Source: CAD feature listing. Evaluate the final solid. Frame: model axes, mm. A direction names the side the tool comes from. Give positions to 0.01 mm unless a question says otherwise; leave off trailing zeros. Order: outer loops, then holes, each group sorted by start corner. A loop starts at its lowest first (then second) coordinate and runs counter-clockwise, first axis right, second up. Notation, with made-up numbers: M 23.25,5.5 L 37.25,5.5 A23 ccw 37.25,29.5 Z; hole C 14.25,9.5 d9. An arc over 180 degrees is marked long. Answer in a Markdown table with one row per item. Add a question column.
(1) Section query A-A, the plane z = 2. Return loops of the section in (x, y), plus the area to 3 significant figures.
(2) Section query B-B, the plane z = 5. Return loops of the section in (x, y).
(3) Set-up query: faces 1 (the face through (11.16, 9.36, 2.23)), 2 (the face through (-11, -11, 3.5)), 3 (the face through (11.33, 9.87, 0.49)), 4 (the face through (0, -14, 0)). Return all of +Z, -Z, +X, -X, +Y, -Y with unobstructed straight access to the full face (end or side cutting, diameter ignored); none if empty.
(4) Mould query, pull axis X, two halves, no side actions, for faces 5 (the face through (-16, -11, 9.5)), 6 (the face through (20.03, 6.31, 5.19)), 7 (the face through (-11.16, -9.36, 2.23)). Classes: pulls with the +X half, pulls with the -X half, needs draft (parallel to the pull), parting line crosses it, or undercut.
(5) Pin query (flat end, axial travel): P1, Ø4, axis at x = -3.5, y = 16, coming from the +Z side; P2, Ø1.8, axis at x = -2, z = 5, coming from the +Y side; P3, Ø3, axis at x = -7.5, z = 6, coming from the +Y side; P4, Ø19, axis at x = -10.5, y = -10, coming from the +Z side. Return the tip coordinate at first contact, or that it passes through.
(6) Material intervals for line 1 along Y through (x, z) = (0, 8.15); line 2 along Y through (x, z) = (-8, 8.25); line 3 along X through (y, z) = (-3, 9.25), sorted ascending.
from build123d import *

# Parameters (mm, degrees)
F0_R         = 21
F1_DEPTH     = 3
F2_R         = 21
F3_DEPTH     = 0.5
F4_R         = 21
F5_DEPTH     = 3.5
F6_R         = 21
F6_R_2       = 19
F7_DEPTH     = 2.5
F8_SIZE      = 1
F9_T6_DEPTH  = 12.3424053326
F9_T11_DEPTH = 19.8242698458
F9_T17_DEPTH = 12.3424053326
F9_T20_ANGLE = 104.7950367117
F9_T24_DEPTH = 12.3424053326
F9_T29_DEPTH = 19.8242698458
F9_T35_DEPTH = 12.3424053326
F9_T38_ANGLE = 104.7950367117
F9_T43_DEPTH = 12.3424053326
F9_T47_DEPTH = 19.8242698458
F9_T54_DEPTH = 19.8242698458
F9_T58_DEPTH = 12.3424053326
F9_T65_DEPTH = 12.3424053326
F9_T69_DEPTH = 19.8242698458
F9_T76_DEPTH = 19.8242698458
F9_T80_DEPTH = 12.3424053326


# Not quite as in the source:
# - a fillet or chamfer that OpenCascade refuses, or shapes differently, is made with other operations: its cross-section is extruded or revolved along the edge and cut away or added


with BuildPart() as f1:
    # F0 (on Top) → F1 (new body)
    with BuildSketch(Plane.XY):
        Circle(F0_R)
        with BuildLine():
            Line((-15.0814358373, 6.3381057238), (-7.340451935, 12.3))
            Line((-7.340451935, 12.3), (7.340451935, 12.3))
            Line((7.340451935, 12.3), (15.0814358373, 6.3381057238))
            ThreePointArc((15.0814358373, 6.3381057238), (18.2, 0), (15.0814358373, -6.3381057238))
            Line((15.0814358373, -6.3381057238), (7.340451935, -12.3))
            Line((7.340451935, -12.3), (-7.340451935, -12.3))
            Line((-7.340451935, -12.3), (-15.0814358373, -6.3381057238))
            ThreePointArc((-15.0814358373, -6.3381057238), (-18.2, 0), (-15.0814358373, 6.3381057238))
        make_face(mode=Mode.SUBTRACT)
    extrude(amount=F1_DEPTH)

    # F2 (on face) → F3 (join)
    with BuildSketch(Plane.XY.offset(3)):
        Circle(F2_R)
        with BuildLine():
            Line((-15.0814358373, 6.3381057238), (-7.340451935, 12.3))
            Line((-7.340451935, 12.3), (-7.2180848246, 12.3))
            Line((-7.2180848246, 12.3), (-5.5458425084, 14.4712563576))
            ThreePointArc((-5.5458425084, 14.4712563576), (-3.0904049489, 16.4808755163), (0, 17.2))
            ThreePointArc((0, 17.2), (3.0904049489, 16.4808755163), (5.5458425084, 14.4712563576))
            Line((5.5458425084, 14.4712563576), (7.2180848246, 12.3))
            Line((7.2180848246, 12.3), (7.340451935, 12.3))
            Line((7.340451935, 12.3), (15.0814358373, 6.3381057238))
            ThreePointArc((15.0814358373, 6.3381057238), (17.3781434472, 3.5318913702), (18.2, 0))
            ThreePointArc((18.2, 0), (17.3781434472, -3.5318913702), (15.0814358373, -6.3381057238))
            Line((15.0814358373, -6.3381057238), (7.340451935, -12.3))
            Line((7.340451935, -12.3), (7.2180848246, -12.3))
            Line((7.2180848246, -12.3), (5.5458425084, -14.4712563576))
            ThreePointArc((5.5458425084, -14.4712563576), (3.0904049489, -16.4808755163), (0, -17.2))
            ThreePointArc((0, -17.2), (-3.0904049489, -16.4808755163), (-5.5458425084, -14.4712563576))
            Line((-5.5458425084, -14.4712563576), (-7.2180848246, -12.3))
            Line((-7.2180848246, -12.3), (-7.340451935, -12.3))
            Line((-7.340451935, -12.3), (-15.0814358373, -6.3381057238))
            ThreePointArc((-15.0814358373, -6.3381057238), (-17.3781434472, -3.5318913702), (-18.2, 0))
            ThreePointArc((-18.2, 0), (-17.3781434472, 3.5318913702), (-15.0814358373, 6.3381057238))
        make_face(mode=Mode.SUBTRACT)
    extrude(amount=F3_DEPTH)

    # F4 (on face) → F5 (join)
    with BuildSketch(Plane.XY.offset(3.5)):
        Circle(F4_R)
        with BuildLine():
            Line((-15.0814358373, 6.3381057238), (-7.340451935, 12.3))
            Line((-7.340451935, 12.3), (-7.2180848246, 12.3))
            Line((-7.2180848246, 12.3), (-5.5458425084, 14.4712563576))
            ThreePointArc((-5.5458425084, 14.4712563576), (-3.0904049489, 16.4808755163), (0, 17.2))
            ThreePointArc((0, 17.2), (12.8139825122, 12.529911728), (18.2, 0))
            ThreePointArc((18.2, 0), (17.3781434472, -3.5318913702), (15.0814358373, -6.3381057238))
            Line((15.0814358373, -6.3381057238), (7.340451935, -12.3))
            Line((7.340451935, -12.3), (7.2180848246, -12.3))
            Line((7.2180848246, -12.3), (5.5458425084, -14.4712563576))
            ThreePointArc((5.5458425084, -14.4712563576), (3.0904049489, -16.4808755163), (0, -17.2))
            ThreePointArc((0, -17.2), (-12.8139825122, -12.529911728), (-18.2, 0))
            ThreePointArc((-18.2, 0), (-17.3781434472, 3.5318913702), (-15.0814358373, 6.3381057238))
        make_face(mode=Mode.SUBTRACT)
    extrude(amount=F5_DEPTH)

    # F6 (on face) → F7 (join)
    with BuildSketch(Plane.XY.offset(7)):
        Circle(F6_R)
        Circle(F6_R_2, mode=Mode.SUBTRACT)
    extrude(amount=F7_DEPTH)

    # F8
    f8_edges = [f1.edges().sort_by_distance(p)[0] for p in [
        (-21, 0, 0),
    ]]
    chamfer(f8_edges, length=F8_SIZE)

    # F9: chamfer of 1 on 9 edges, made by hand

    # F9_s1 → F9_t2 (revolve, cut)
    with BuildSketch(Plane.XZ):
        Polygon((20.2928932188, 0.2928932188), (19.5857864376, 0), (20, 0), align=None)
    revolve(axis=Axis((0, 0, 0), (0, 0, 1)), mode=Mode.SUBTRACT)


with BuildPart() as f9_tool4:
    # F9_s5 → F9_t6 (new body)
    with BuildSketch(Plane(origin=(-6.4023462265, -4.9309121171, 0), x_dir=(0, 0, 1), z_dir=(0.7922632155, 0.6101794797, 0))):
        Polygon((0, -15.2238306925), (1, -14.2238306925), (0, -14.2238306925), align=None)
    extrude(amount=F9_T6_DEPTH)

    split(bisect_by=Plane.XZ.offset(-12.3), keep=Keep.TOP)


with BuildPart() as f1_1:
    add(f1.part)

    # F9_t3: cut F9_tool4
    add(f9_tool4.part, mode=Mode.SUBTRACT)


with BuildPart() as f9_tool9:
    # F9_s10 → F9_t11 (new body)
    with BuildSketch(Plane.YZ.offset(-9.9121349229)):
        Polygon((13.3, 0), (12.3, 1), (12.3, 0), align=None)
    extrude(amount=F9_T11_DEPTH)

    split(bisect_by=Plane(origin=(-8.6790896108, 11.2690178409, 0), x_dir=(0, 0, 1), z_dir=(0.6101794797, -0.7922632155, 0)), keep=Keep.TOP)

    split(bisect_by=Plane(origin=(8.6790896108, 11.2690178409, 0), x_dir=(0, 0, 1), z_dir=(-0.6101794797, -0.7922632155, 0)), keep=Keep.TOP)


with BuildPart() as f1_2:
    add(f1_1.part)

    # F9_t8: cut F9_tool9
    add(f9_tool9.part, mode=Mode.SUBTRACT)


with BuildPart() as f9_tool15:
    # F9_s16 → F9_t17 (new body)
    with BuildSketch(Plane(origin=(-3.376087509, 2.6001703465, 0), x_dir=(0, 0, 1), z_dir=(0.7922632155, -0.6101794797, 0))):
        Polygon((0, -15.2238306925), (1, -14.2238306925), (0, -14.2238306925), align=None)
    extrude(amount=F9_T17_DEPTH)

    split(bisect_by=Plane.XZ.offset(-12.3), keep=Keep.TOP)


with BuildPart() as f1_3:
    add(f1_2.part)

    # F9_t14: cut F9_tool15
    add(f9_tool15.part, mode=Mode.SUBTRACT)

    # F9_s19 → F9_t20 (revolve, cut)
    with BuildSketch(Plane(origin=(6.4023462265, -4.9309121171, 0), x_dir=(0, 0, 1), z_dir=(-0.7922632155, 0.6101794797, 0))):
        Polygon((0, 15.2238306925), (1, 14.2238306925), (0, 14.2238306925), align=None)
    revolve(axis=Axis((10.2, 0, 0), (0, 0, -1)), revolution_arc=F9_T20_ANGLE, mode=Mode.SUBTRACT)


with BuildPart() as f9_tool22:
    # F9_s23 → F9_t24 (new body)
    with BuildSketch(Plane(origin=(6.4023462265, 4.9309121171, 0), x_dir=(0, 0, 1), z_dir=(-0.7922632155, -0.6101794797, 0))):
        Polygon((0, -15.2238306925), (1, -14.2238306925), (0, -14.2238306925), align=None)
    extrude(amount=F9_T24_DEPTH)

    split(bisect_by=Plane.XZ.offset(12.3), keep=Keep.BOTTOM)


with BuildPart() as f1_4:
    add(f1_3.part)

    # F9_t21: cut F9_tool22
    add(f9_tool22.part, mode=Mode.SUBTRACT)


with BuildPart() as f9_tool27:
    # F9_s28 → F9_t29 (new body)
    with BuildSketch(Plane.YZ.offset(9.9121349229)):
        Polygon((-13.3, 0), (-12.3, 1), (-12.3, 0), align=None)
    extrude(amount=-F9_T29_DEPTH)

    split(bisect_by=Plane(origin=(8.6790896108, -11.2690178409, 0), x_dir=(0, 0, 1), z_dir=(-0.6101794797, 0.7922632155, 0)), keep=Keep.TOP)

    split(bisect_by=Plane(origin=(-8.6790896108, -11.2690178409, 0), x_dir=(0, 0, 1), z_dir=(0.6101794797, 0.7922632155, 0)), keep=Keep.TOP)


with BuildPart() as f1_5:
    add(f1_4.part)

    # F9_t26: cut F9_tool27
    add(f9_tool27.part, mode=Mode.SUBTRACT)


with BuildPart() as f9_tool33:
    # F9_s34 → F9_t35 (new body)
    with BuildSketch(Plane(origin=(3.376087509, -2.6001703465, 0), x_dir=(0, 0, 1), z_dir=(-0.7922632155, 0.6101794797, 0))):
        Polygon((0, -15.2238306925), (1, -14.2238306925), (0, -14.2238306925), align=None)
    extrude(amount=F9_T35_DEPTH)

    split(bisect_by=Plane.XZ.offset(12.3), keep=Keep.BOTTOM)


with BuildPart() as f1_6:
    add(f1_5.part)

    # F9_t32: cut F9_tool33
    add(f9_tool33.part, mode=Mode.SUBTRACT)

    # F9_s37 → F9_t38 (revolve, cut)
    with BuildSketch(Plane(origin=(-6.4023462265, 4.9309121171, 0), x_dir=(0, 0, 1), z_dir=(0.7922632155, -0.6101794797, 0))):
        Polygon((0, 15.2238306925), (1, 14.2238306925), (0, 14.2238306925), align=None)
    revolve(axis=Axis((-10.2, 0, 0), (0, 0, -1)), revolution_arc=F9_T38_ANGLE, mode=Mode.SUBTRACT)


with BuildPart() as f9_tool41:
    # F9_s42 → F9_t43 (new body)
    with BuildSketch(Plane(origin=(-6.4023462265, -4.9309121171, 0), x_dir=(0, 0, 1), z_dir=(0.7922632155, 0.6101794797, 0))):
        Polygon((0, -15.2238306925), (1, -14.2238306925), (0, -14.2238306925), align=None)
    extrude(amount=F9_T43_DEPTH)

    split(bisect_by=Plane.XZ.offset(-12.3), keep=Keep.BOTTOM)


with BuildPart() as f9_tool45:
    # F9_s46 → F9_t47 (new body)
    with BuildSketch(Plane.YZ.offset(-9.9121349229)):
        Polygon((13.3, 0), (12.3, 1), (12.3, 0), align=None)
    extrude(amount=F9_T47_DEPTH)

    split(bisect_by=Plane(origin=(-8.6790896108, 11.2690178409, 0), x_dir=(0, 0, 1), z_dir=(-0.6101794797, 0.7922632155, 0)), keep=Keep.TOP)


with BuildPart() as f9_tool41_1:
    add(f9_tool41.part)

    # F9_t49: intersect F9_tool45
    add(f9_tool45.part, mode=Mode.INTERSECT)


with BuildPart() as f1_7:
    add(f1_6.part)

    # F9_t39: cut F9_tool41
    add(f9_tool41_1.part, mode=Mode.SUBTRACT)


with BuildPart() as f9_tool52:
    # F9_s53 → F9_t54 (new body)
    with BuildSketch(Plane.YZ.offset(-9.9121349229)):
        Polygon((13.3, 0), (12.3, 1), (12.3, 0), align=None)
    extrude(amount=F9_T54_DEPTH)

    split(bisect_by=Plane(origin=(8.6790896108, 11.2690178409, 0), x_dir=(0, 0, 1), z_dir=(0.6101794797, 0.7922632155, 0)), keep=Keep.TOP)


with BuildPart() as f9_tool56:
    # F9_s57 → F9_t58 (new body)
    with BuildSketch(Plane(origin=(-3.376087509, 2.6001703465, 0), x_dir=(0, 0, 1), z_dir=(0.7922632155, -0.6101794797, 0))):
        Polygon((0, -15.2238306925), (1, -14.2238306925), (0, -14.2238306925), align=None)
    extrude(amount=F9_T58_DEPTH)

    split(bisect_by=Plane.XZ.offset(-12.3), keep=Keep.BOTTOM)


with BuildPart() as f9_tool52_1:
    add(f9_tool52.part)

    # F9_t60: intersect F9_tool56
    add(f9_tool56.part, mode=Mode.INTERSECT)


with BuildPart() as f1_8:
    add(f1_7.part)

    # F9_t50: cut F9_tool52
    add(f9_tool52_1.part, mode=Mode.SUBTRACT)


with BuildPart() as f9_tool63:
    # F9_s64 → F9_t65 (new body)
    with BuildSketch(Plane(origin=(6.4023462265, 4.9309121171, 0), x_dir=(0, 0, 1), z_dir=(-0.7922632155, -0.6101794797, 0))):
        Polygon((0, -15.2238306925), (1, -14.2238306925), (0, -14.2238306925), align=None)
    extrude(amount=F9_T65_DEPTH)

    split(bisect_by=Plane.XZ.offset(12.3), keep=Keep.TOP)


with BuildPart() as f9_tool67:
    # F9_s68 → F9_t69 (new body)
    with BuildSketch(Plane.YZ.offset(9.9121349229)):
        Polygon((-13.3, 0), (-12.3, 1), (-12.3, 0), align=None)
    extrude(amount=-F9_T69_DEPTH)

    split(bisect_by=Plane(origin=(8.6790896108, -11.2690178409, 0), x_dir=(0, 0, 1), z_dir=(0.6101794797, -0.7922632155, 0)), keep=Keep.TOP)


with BuildPart() as f9_tool63_1:
    add(f9_tool63.part)

    # F9_t71: intersect F9_tool67
    add(f9_tool67.part, mode=Mode.INTERSECT)


with BuildPart() as f1_9:
    add(f1_8.part)

    # F9_t61: cut F9_tool63
    add(f9_tool63_1.part, mode=Mode.SUBTRACT)


with BuildPart() as f9_tool74:
    # F9_s75 → F9_t76 (new body)
    with BuildSketch(Plane.YZ.offset(9.9121349229)):
        Polygon((-13.3, 0), (-12.3, 1), (-12.3, 0), align=None)
    extrude(amount=-F9_T76_DEPTH)

    split(bisect_by=Plane(origin=(-8.6790896108, -11.2690178409, 0), x_dir=(0, 0, 1), z_dir=(-0.6101794797, -0.7922632155, 0)), keep=Keep.TOP)


with BuildPart() as f9_tool78:
    # F9_s79 → F9_t80 (new body)
    with BuildSketch(Plane(origin=(3.376087509, -2.6001703465, 0), x_dir=(0, 0, 1), z_dir=(-0.7922632155, 0.6101794797, 0))):
        Polygon((0, -15.2238306925), (1, -14.2238306925), (0, -14.2238306925), align=None)
    extrude(amount=F9_T80_DEPTH)

    split(bisect_by=Plane.XZ.offset(12.3), keep=Keep.TOP)


with BuildPart() as f9_tool74_1:
    add(f9_tool74.part)

    # F9_t82: intersect F9_tool78
    add(f9_tool78.part, mode=Mode.INTERSECT)


with BuildPart() as f1_10:
    add(f1_9.part)

    # F9_t72: cut F9_tool74
    add(f9_tool74_1.part, mode=Mode.SUBTRACT)


solid = f1_10.part
Values follow:
| question | item | result |
|---|---|---|
| 1 | outline | C 0,0 d42; hole M -15.08,-6.34 L -7.34,-12.3 L 7.34,-12.3 L 15.08,-6.34 A8 ccw 15.08,6.34 L 7.34,12.3 L -7.34,12.3 L -15.08,6.34 A8 ccw Z |
| 1 | area | 681 mm² |
| 2 | outline | C 0,0 d42; hole M -18.2,0 A17.2 ccw 0,-17.2 A7 ccw 5.55,-14.47 L 7.22,-12.3 L 7.34,-12.3 L 15.08,-6.34 A8 ccw 18.2,0 A17.2 ccw 0,17.2 A7 ccw -5.55,14.47 L -7.22,12.3 L -7.34,12.3 L -15.08,6.34 A8 ccw Z |
| 3 | face 1 | +Z, -Z |
| 3 | face 2 | +Z |
| 3 | face 3 | -Z |
| 3 | face 4 | -Z, +X, -X, +Y, -Y |
| 4 | face 5 | needs draft |
| 4 | face 6 | parting line crosses it |
| 4 | face 7 | undercut |
| 5 | P1 | stops at z = 7 |
| 5 | P2 | stops at y = 20.97 |
| 5 | P3 | stops at y = 20.12 |
| 5 | P4 | stops at z = 9.5 |
| 6 | line 1 | y = -21 to -19, 19 to 21 |
| 6 | line 2 | y = -19.42 to -17.23, 17.23 to 19.42 |
| 6 | line 3 | x = -20.78 to -18.76, 18.76 to 20.78 |
